Design review of the part built by this model. Coordinates are the model's own, in mm. Coordinates: 2 decimals unless noted, no trailing zeros. Write each loop counter-clockwise with the first axis right and the second up, starting at its lowest first coordinate (ties: lowest second). Pieces come first, ordered by that corner, then holes. Notation, with made-up numbers: (27.25, 36.25) - (54.25, 36.25) arc R8 ccw to (54.25, 47.25) - close; hole circle Ø3 at (53, 49). An arc over 180 degrees is marked (long way). One line per item, written item: value.
from build123d import *

# Parameters (mm, degrees)
SKETCH1_W           = 129.4
SKETCH1_H           = 79.9
BOSS_EXTRUDE1_DEPTH = 4
FILLET1_R           = 3
CUT_EXTRUDE1_DEPTH  = 10
SKETCH3_R           = 10.5
SKETCH3_R_2         = 1.6
SKETCH3_R_3         = 16.5
CUT_EXTRUDE2_DEPTH  = 10
SKETCH4_R           = 1.6
CUT_EXTRUDE3_DEPTH  = 10
SKETCH5_W           = 18
SKETCH5_H           = 32
SKETCH5_W_2         = 17
CUT_EXTRUDE4_DEPTH  = 10
SKETCH6_W           = 5
SKETCH6_H           = 63.9
CUT_EXTRUDE5_DEPTH  = 10
FILLET2_R           = 2
SKETCH7_R           = 1.6
CUT_EXTRUDE6_DEPTH  = 10
FILLET3_R           = 3


with BuildPart() as part:
    # Sketch1 → Boss-Extrude1 (new body)
    with BuildSketch(Plane(origin=(0, 0, 0), x_dir=(1, 0, 0), z_dir=(0, 1, 0))):
        with Locations((64.7, 39.95)):
            Rectangle(SKETCH1_W, SKETCH1_H)
    extrude(amount=BOSS_EXTRUDE1_DEPTH)

    # Fillet1
    fillet1_edges = [part.edges().sort_by_distance(p)[0] for p in [
        (0, 2, -79.9),
        (129.4, 2, -79.9),
        (129.4, 2, 0),
        (0, 2, 0),
    ]]
    fillet(fillet1_edges, radius=FILLET1_R)

    # Sketch2 → Cut-Extrude1 (cut)
    with BuildSketch(Plane(origin=(0, 4, 0), x_dir=(1, 0, 0), z_dir=(0, 1, 0))):
        Polygon((5, 4.55), (26, 4.55), (26, 54.65), (55.1, 54.65), (55.1, 75.65), (5, 75.65), (5, 40), align=None)
    extrude(amount=-CUT_EXTRUDE1_DEPTH, mode=Mode.SUBTRACT)

    # Sketch3 → Cut-Extrude2 (cut)
    with BuildSketch(Plane(origin=(0, 4, 0), x_dir=(1, 0, 0), z_dir=(0, 1, 0))):
        with Locations((91.05, 59.55)):
            Circle(SKETCH3_R)
        with Locations((83.05, 73.3)):
            Circle(SKETCH3_R_2)
        with Locations((99.05, 73.3)):
            Circle(SKETCH3_R_2)
        with Locations((99.05, 45.8)):
            Circle(SKETCH3_R_2)
        with Locations((83.05, 45.8)):
            Circle(SKETCH3_R_2)
        with Locations((41.4, 36.5)):
            Circle(SKETCH3_R_2)
        with Locations((73.4, 36.5)):
            Circle(SKETCH3_R_2)
        with Locations((86, 36.5)):
            Circle(SKETCH3_R_2)
        with Locations((118, 36.5)):
            Circle(SKETCH3_R_2)
        with Locations((102, 20.5)):
            Circle(SKETCH3_R_3)
        with Locations((57.4, 20.5)):
            Circle(SKETCH3_R_3)
        with Locations((41.4, 4.5)):
            Circle(SKETCH3_R_2)
        with Locations((73.4, 4.5)):
            Circle(SKETCH3_R_2)
        with Locations((86, 4.5)):
            Circle(SKETCH3_R_2)
        with Locations((118, 4.5)):
            Circle(SKETCH3_R_2)
    extrude(amount=-CUT_EXTRUDE2_DEPTH, mode=Mode.SUBTRACT)

    # Sketch4 → Cut-Extrude3 (cut)
    with BuildSketch(Plane(origin=(0, 4, 0), x_dir=(1, 0, 0), z_dir=(0, 1, 0))):
        with Locations((125.5, 4)):
            Circle(SKETCH4_R)
        with Locations((125.5, 76)):
            Circle(SKETCH4_R)
        with Locations((29.9, 50.55)):
            Circle(SKETCH4_R)
        with Locations((29.9, 4)):
            Circle(SKETCH4_R)
    extrude(amount=-CUT_EXTRUDE3_DEPTH, mode=Mode.SUBTRACT)

    # Sketch5 → Cut-Extrude4 (cut)
    with BuildSketch(Plane(origin=(0, 4, 0), x_dir=(1, 0, 0), z_dir=(0, 1, 0))):
        with Locations((68.35, 59.65)):
            Rectangle(SKETCH5_W, SKETCH5_H)
        with Locations((113.25, 59.65)):
            Rectangle(SKETCH5_W_2, SKETCH5_H)
    extrude(amount=-CUT_EXTRUDE4_DEPTH, mode=Mode.SUBTRACT)

    # Sketch6 → Cut-Extrude5 (cut)
    with BuildSketch(Plane(origin=(0, 4, 0), x_dir=(1, 0, 0), z_dir=(0, 1, 0))):
        with Locations((126.9, 39.95)):
            Rectangle(SKETCH6_W, SKETCH6_H)
    extrude(amount=-CUT_EXTRUDE5_DEPTH, mode=Mode.SUBTRACT)

    # Fillet2
    fillet2_edges = [part.edges().sort_by_distance(p)[0] for p in [
        (129.4, 2, -71.9),
        (129.4, 2, -8),
        (124.4, 2, -8),
        (124.4, 2, -71.9),
    ]]
    fillet(fillet2_edges, radius=FILLET2_R)

    # Sketch7 → Cut-Extrude6 (cut)
    with BuildSketch(Plane(origin=(0, 0, 0), x_dir=(-1, 0, 0), z_dir=(0, -1, 0))):
        with Locations((-2.5, 17.775)):
            Circle(SKETCH7_R)
        with Locations((-2.5, 62.225)):
            Circle(SKETCH7_R)
    extrude(amount=-CUT_EXTRUDE6_DEPTH, mode=Mode.SUBTRACT)

    # Fillet3
    fillet3_edges = [part.edges().sort_by_distance(p)[0] for p in [
        (77.35, 2, -43.65),
        (59.35, 2, -43.65),
        (59.35, 2, -75.65),
        (77.35, 2, -75.65),
        (121.75, 2, -75.65),
        (121.75, 2, -43.65),
        (104.75, 2, -43.65),
        (104.75, 2, -75.65),
    ]]
    fillet(fillet3_edges, radius=FILLET3_R)


solid = part.part
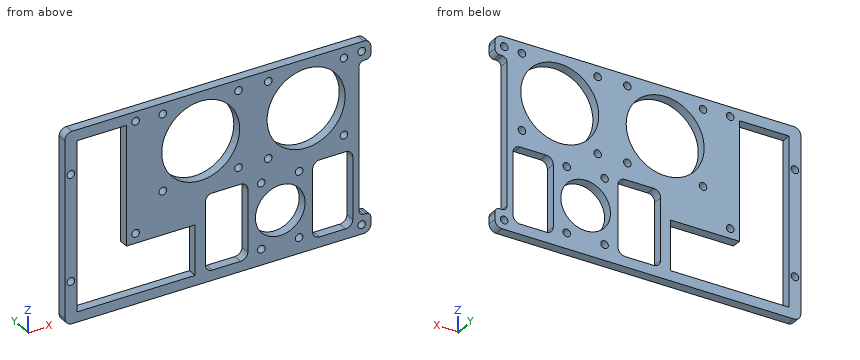
1. Insertion check: pin 1 Ø2 at (x, z) = (103.5, -57) entering from -Y; pin 2 Ø0.8 at (x, y) = (127, 1) entering from +Z; pin 3 Ø2 at (y, z) = (1.5, -63) entering from +X. Each pin has a flat end and moves straight along its axis. Give the tip position at first contact, or say it passes through.
Answer block:
pin 1: stops at y = 0
pin 2: stops at z = -0.01
pin 3: stops at x = 124.4
2. Wall thickness on line 1 along Z through (x, y) = (102, 2.5); line 2 along Z through (x, y) = (48.5, 1.15); line 3 along X through (y, z) = (1, -73.3): over which ranges is each line inside the solid? List them lowest first.
Answer block:
line 1: z = -79.9 to -37, -4 to 0
line 2: z = -79.9 to -75.65, -54.65 to -34.39, -6.61 to 0
line 3: x = 0 to 5, 55.1 to 59.42, 77.28 to 81.45, 84.65 to 97.45, 100.65 to 104.82, 121.68 to 129.31
3. Consider section B-B, the plane z = -56.5. Write out the cut boundary in (x, y).
Answer block:
outline: (0, 0) - (5, 0) - (5, 4) - (0, 4) - close; (55.1, 0) - (59.35, 0) - (59.35, 4) - (55.1, 4) - close; (77.35, 0) - (81, 0) - (81, 4) - (77.35, 4) - close; (101.1, 0) - (104.75, 0) - (104.75, 4) - (101.1, 4) - close; (121.75, 0) - (124.4, 0) - (124.4, 4) - (121.75, 4) - close
4. Consider section D-D, the plane x = 50. Write out the cut boundary in (y, z), then the cut area to 3 significant figures.
Answer block:
outline: (0, -79.9) - (4, -79.9) - (4, -75.65) - (0, -75.65) - close; (0, -54.65) - (4, -54.65) - (4, -35.25) - (0, -35.25) - close; (0, -5.75) - (4, -5.75) - (4, 0) - (0, 0) - close
area: 118 mm^2
5. Consider section A-A, the plane x = 92. Write out the cut boundary in (y, z).
Answer block:
outline: (0, -79.9) - (4, -79.9) - (4, -70.01) - (0, -70.01) - close; (0, -49.09) - (4, -49.09) - (4, -33.62) - (0, -33.62) - close; (0, -7.38) - (4, -7.38) - (4, 0) - (0, 0) - close
6. Consider section C-C, the plane z = -24.5. Write out the cut boundary in (x, y), then the cut area to 3 significant figures.
Answer block:
outline: (0, 0) - (5, 0) - (5, 4) - (0, 4) - close; (26, 0) - (41.39, 0) - (41.39, 4) - (26, 4) - close; (73.41, 0) - (85.99, 0) - (85.99, 4) - (73.41, 4) - close; (118.01, 0) - (124.4, 0) - (124.4, 4) - (118.01, 4) - close
area: 157 mm^2
